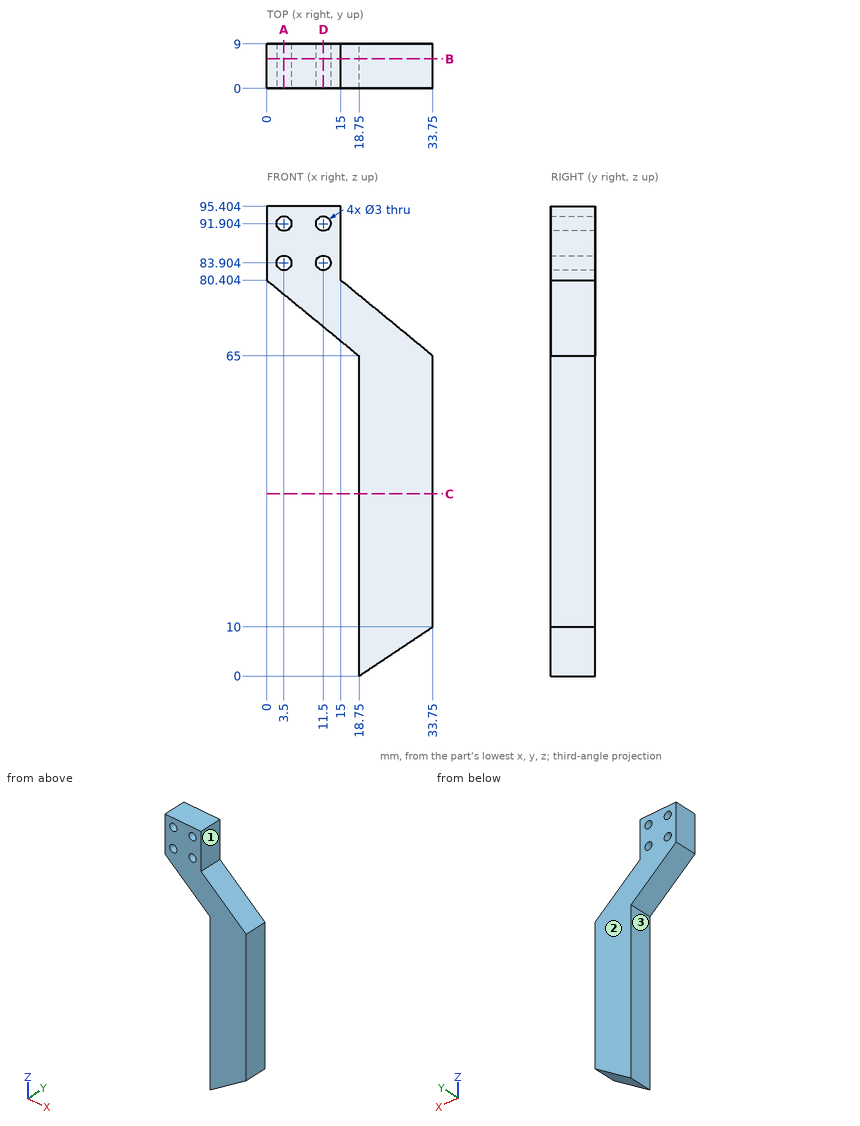
For this review, use the dimensioned drawing (mm, ordinates from the lowest corner) and the shaded views. A direction names the side the tool comes from. Coordinates: 2 decimals unless noted, no trailing zeros. Order: outer loops, then holes, each group sorted by start corner. A loop starts at its lowest first (then second) coordinate and runs counter-clockwise, first axis right, second up. Notation, with made-up numbers: (19.5, 79.25) -> (24.5, 79.25) arc R37 ccw to (24.5, 117.25) -> close; hole circle Ø1 at (67, -6). An arc over 180 degrees is marked (long way). One line per item, written item: value. Start each with the question number.
Q1. Tool access review of the marked faces 1, 2 and 3: name each direction out of +Z, -Z, +X, -X, +Y, -Y from which nothing blocks a thin tool from reaching the whole face with its end or side.
Q2. For probe 1 along X at (y, z) = (8.25, 12); probe 2 along X at (y, z) = (8.25, 90); probe 3 along Z at (x, y) = (13.5, 1.75) (1 decimal), list the stretches that pass through material, from the lowest coordinate up.
Q3. Take a section at D-D, the plane x = 11.5. State the section outline as (y, z) points.
Q4. Take a section at B-B, the plane y = 6. State the section outline as (x, z) points, then the cut area to 3 significant figures.
Q5. Take a section at C-C, the plane z = 37. State the section outline as (x, y) points, then the cut area to 3 significant figures.
Q6. Take a section at A-A, the plane x = 3.5. State the section outline as (y, z) points, then the cut area to 3 significant figures.
Q7. Insertion check: pin 1 Ø4 at (x, z) = (3.5, 83.9) entering from -Y; pin 2 Ø2.5 at (y, z) = (4, 90) entering from +X; pin 3 Ø1 at (y, z) = (4.5, 22.5) entering from -X. Each pin has a flat end and moves straight along its axis. Give the tip position at first contact, or say it passes through.
Values follow:
1. face 1: +Z, +X, +Y, -Y
1. face 2: +Z, -Z, +X, -X, +Y
1. face 3: -Z, -X, +Y, -Y
2. probe 1: x = 18.75 to 33.75
2. probe 2: x = 0 to 15
2. probe 3: z = 69.3 to 95.4
3. outline: (0, 70.96) -> (9, 70.96) -> (9, 82.4) -> (0, 82.4) -> close; (0, 85.4) -> (9, 85.4) -> (9, 90.4) -> (0, 90.4) -> close; (0, 93.4) -> (9, 93.4) -> (9, 95.4) -> (0, 95.4) -> close
4. outline: (0, 80.4) -> (18.75, 65) -> (18.75, 0) -> (33.75, 10) -> (33.75, 65) -> (15, 80.4) -> (15, 95.4) -> (0, 95.4) -> close; hole circle Ø3 at (3.5, 83.9); hole circle Ø3 at (3.5, 91.9); hole circle Ø3 at (11.5, 83.9); hole circle Ø3 at (11.5, 91.9)
4. area: 1,330 mm2
5. outline: (18.75, 0) -> (33.75, 0) -> (33.75, 9) -> (18.75, 9) -> close
5. area: 135 mm2
6. outline: (0, 77.53) -> (9, 77.53) -> (9, 82.4) -> (0, 82.4) -> close; (0, 85.4) -> (9, 85.4) -> (9, 90.4) -> (0, 90.4) -> close; (0, 93.4) -> (9, 93.4) -> (9, 95.4) -> (0, 95.4) -> close
6. area: 107 mm2
7. pin 1: stops at y = 0
7. pin 2: stops at x = 15
7. pin 3: stops at x = 18.75
